Verification items for this drawing (mm, ordinates from the low corner). Round coordinates to 2 decimals unless told otherwise and drop trailing zeros. Write each loop counter-clockwise with the first axis right and the second up, starting at its lowest first coordinate (ties: lowest second). Pieces come first, ordered by that corner, then holes. Notation, with made-up numbers: (61, 23.25) - (103, 23.25) arc R25 ccw to (103, 52.25) - close; hole circle Ø1 at (-17, -12.75). An arc over 180 degrees is marked (long way). One line per question, with ' | ' between items. Start each with the question number.
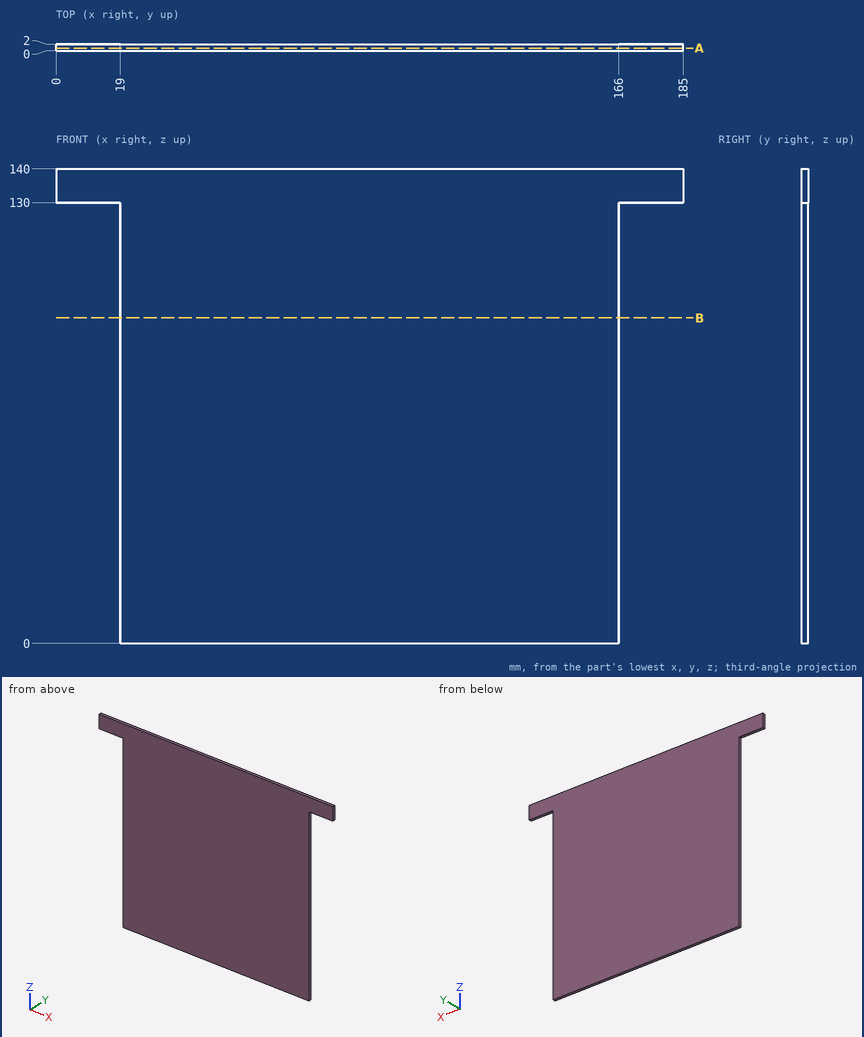
Q1. Go/stop test with flat-tipped pins: P1, Ø0.6, axis at y = 1, z = 48.5, coming from the +X side; P2, Ø1, axis at y = 2, z = 50.5, coming from the -X side. Record where each tip stops, or that it passes through.
Q2. Section check A-A, the plane y = 0.75. Record the cut outline in (x, z).
Q3. Thickness scan on line 1 (Z direction, x = 175, y = 1.2); line 2 (X direction, y = 0.45, z = 70). Record the ranges inside material, lowest first.
Q4. Section check B-B, the plane z = 96. Record the cut outline in (x, y).
Result sheet:
1) P1: x = 166 | P2: x = 19
2) outline: (0, 130) - (19, 130) - (19, 0) - (166, 0) - (166, 130) - (185, 130) - (185, 140) - (0, 140) - close
3) line 1: 130 to 140 | line 2: 19 to 166
4) outline: (19, 0) - (166, 0) - (166, 2) - (19, 2) - close
